from build123d import *

# Parameters (mm, degrees)
SKETCH_1_R               = 57.8
SKETCH_1_R_2             = 48
EXTRUDE_1_DEPTH          = 41.4
SKETCH_2_R               = 2.75
CUT_EXTRUDE_1_DEPTH      = 92.627725062
PATTERN_CIRCULAR_1_COUNT = 12
SKETCH_3_R               = 2.5
CUT_EXTRUDE_2_DEPTH      = 92.627725062
PATTERN_CIRCULAR_2_COUNT = 6


with BuildPart() as part:
    # 草图1 → 凸台-拉伸1 (new body)
    with BuildSketch(Plane(origin=(0, 0, 0), x_dir=(1, 0, 0), z_dir=(0, 1, 0))):
        with Locations(Location((0, 0, 0), (0, 0, 270))):
            Circle(SKETCH_1_R)
        with Locations(Location((0, 0, 0), (0, 0, 270))):
            Circle(SKETCH_1_R_2, mode=Mode.SUBTRACT)
    extrude(amount=EXTRUDE_1_DEPTH)

    # 草图2 → 切除-拉伸1 (cut, symmetric)
    with BuildSketch(Plane(origin=(0, 41.4, 0), x_dir=(1, 0, 0), z_dir=(0, 1, 0))):
        with Locations(Location((0, 54, 0), (0, 0, 270))):
            Circle(SKETCH_2_R)
    cut_extrude_1 = extrude(amount=CUT_EXTRUDE_1_DEPTH, both=True, mode=Mode.SUBTRACT)

    # 阵列(圆周)1: 切除-拉伸1 ×12 about axis
    pattern_circular_1_axis = Axis((0, 0, 0), (0, 1, 0))
    for i in range(1, PATTERN_CIRCULAR_1_COUNT):
        add(cut_extrude_1.rotate(pattern_circular_1_axis, i * 360 / PATTERN_CIRCULAR_1_COUNT), mode=Mode.SUBTRACT)

    # 草图3 → 切除-拉伸2 (cut, through all)
    with BuildSketch(Plane(origin=(0, 0, 0), x_dir=(0.7071067811865477, 0, 0.7071067811865475), z_dir=(-0.7071067811865475, 0, 0.7071067811865477))):
        with Locations((0, 2.5)):
            Circle(SKETCH_3_R)
        with BuildLine():
            Line((2.5, 0), (2.5, 2.5))
            ThreePointArc((2.5, 2.5), (1.767766953, 0.732233047), (0, 0))
            Line((0, 0), (2.5, 0))
        make_face()
        with BuildLine():
            ThreePointArc((0, 0), (-1.767766953, 0.732233047), (-2.5, 2.5))
            Line((-2.5, 2.5), (-2.5, 0))
            Line((-2.5, 0), (0, 0))
        make_face()
    cut_extrude_2 = extrude(amount=-CUT_EXTRUDE_2_DEPTH, mode=Mode.SUBTRACT)

    # 阵列(圆周)2: 切除-拉伸2 ×6 about axis
    pattern_circular_2_axis = Axis((0, 0, 0), (0, 1, 0))
    for i in range(1, PATTERN_CIRCULAR_2_COUNT):
        add(cut_extrude_2.rotate(pattern_circular_2_axis, i * 360 / PATTERN_CIRCULAR_2_COUNT), mode=Mode.SUBTRACT)


solid = part.part
Build history of the part. All positions in model axes, mm. A direction names the side the tool comes from. Coordinates: 2 decimals unless noted, no trailing zeros. Order: outer loops, then holes, each group sorted by start corner. A loop starts at its lowest first (then second) coordinate and runs counter-clockwise, first axis right, second up. Notation, with made-up numbers: (21, 76) -> (74, 76) arc R26 ccw to (74, 91) -> close; hole circle Ø9 at (0.25, 55.25). An arc over 180 degrees is marked (long way). One line per item, written item: value.
(1) Slice it at A-A, the plane z = 0. List the corners of the cut face in (x, y).
Checked values:
outline: (-57.8, 0) -> (-56.75, 0) -> (-56.75, 41.4) -> (-57.8, 41.4) -> close; (-51.25, 0) -> (-48, 0) -> (-48, 41.4) -> (-51.25, 41.4) -> close; (48, 0) -> (51.25, 0) -> (51.25, 41.4) -> (48, 41.4) -> close; (56.75, 0) -> (57.8, 0) -> (57.8, 41.4) -> (56.75, 41.4) -> close
(2) Mould opens along X. For faces 3 (the cylindrical face through (-24.82, 20.99, 45.09)), 4 (the flat face through (-50.327, 1.233, -16.073)), 5 (the flat face through (49, 0, -14)) say: pulls with the +X half, pulls with the -X half, needs draft (parallel to the pull), parting line crosses it, or undercut.
Checked values:
face 3: undercut
face 4: pulls with the -X half
face 5: needs draft
(3) Slice it at B-B, the plane x = -27. List the corners of the cut face in (y, z), plus the area to 3 significant figures.
Checked values:
outline: (0, -51.11) -> (41.4, -51.11) -> (41.4, -49.52) -> (0, -49.52) -> close; (0, -44.02) -> (41.4, -44.02) -> (41.4, -39.69) -> (0, -39.69) -> close; (0, 39.69) -> (41.4, 39.69) -> (41.4, 44.02) -> (0, 44.02) -> close; (0, 49.52) -> (41.4, 49.52) -> (41.4, 51.11) -> (0, 51.11) -> close
area: 490 mm2
(4) Tool access for faces 1 (the flat face through (-36, 0, -37)), 2 (the flat face through (-35.547, 1.267, 39.083)): list every direction of +Z, -Z, +X, -X, +Y, -Y with a clear straight run to the whole face (end or side of a thin tool).
Checked values:
face 1: +Z, -Z, +X, -X, -Y
face 2: -Y
(5) Slice it at C-C, the plane y = 15.5. Count the separate pieces of the cut face and the enclosed holes in it, plus the area to 3 significant figures.
Checked values:
separate pieces: 1
enclosed holes: 13
area: 2,970 mm2
(6) Probe line 1 (Z direction, x = -27, y = 10); line 2 (Z direction, x = 1, y = 40). List the from-to ranges inside material, lowest first. Write a range as [from, to].
Checked values:
line 1: [-51.11, -49.52], [-44.02, -39.69], [39.69, 44.02], [49.52, 51.11]
line 2: [-57.79, -56.56], [-51.44, -47.99], [47.99, 51.44], [56.56, 57.79]
(7) Drop flat-ended pins along their axis: pin 1 Ø12 at (y, z) = (24, -14.5) entering from -X; pin 2 Ø5 at (y, z) = (29.5, -29.5) entering from -X; pin 3 Ø2 at (y, z) = (10, 33) entering from -X. Give the stop position or say it passes through.
Checked values:
pin 1: x = -57.17
pin 2: x = -51.11
pin 3: x = -48.13
